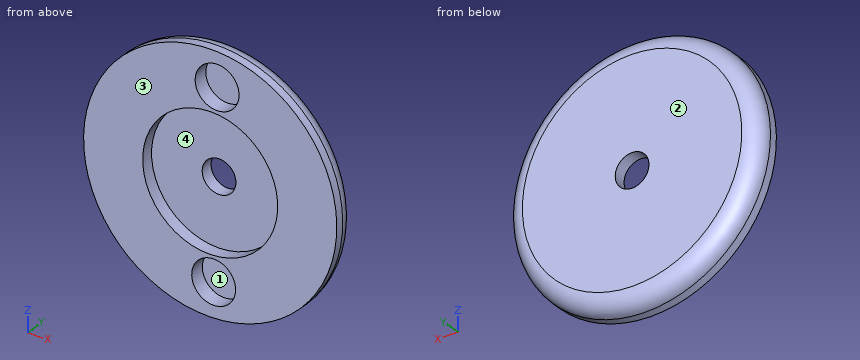
```python
from build123d import *

# Parameters (mm, degrees)
SKETCH2_W          = 15
SKETCH2_H          = 3
SKETCH3_R          = 8
CUT_EXTRUDE1_DEPTH = 1.5
CUT_EXTRUDE2_DEPTH = 1.5
SKETCH5_R          = 2.6
CUT_EXTRUDE3_DEPTH = 1.8
FILLET1_R          = 2


with BuildPart() as part:
    # Sketch2 → Revolve1 (revolve)
    with BuildSketch(Plane.XY, mode=Mode.PRIVATE) as revolve1_sk:
        with Locations((7.5, 1.5)):
            Rectangle(SKETCH2_W, SKETCH2_H)
    revolve(revolve1_sk.sketch.rotate(Axis((0, 0, 0), (0, 1, 0)), 90), axis=Axis((0, 0, 0), (0, 1, 0)))

    # Sketch3 → Cut-Extrude1 (cut)
    with BuildSketch(Plane.XZ):
        with Locations(Location((0, 0, 0), (0, 0, 270))):
            Circle(SKETCH3_R)
    extrude(amount=-CUT_EXTRUDE1_DEPTH, mode=Mode.SUBTRACT)

    # Sketch4 → Cut-Extrude2 (cut)
    with BuildSketch(Plane.XZ.offset(-1.5)):
        with BuildLine():
            ThreePointArc((0, -2), (2, 0), (0, 2))
            ThreePointArc((0, 2), (-2, 0), (0, -2))
        make_face()
    extrude(amount=-CUT_EXTRUDE2_DEPTH, mode=Mode.SUBTRACT)

    # Sketch5 → Cut-Extrude3 (cut)
    with BuildSketch(Plane.XZ):
        with Locations(Location((0.41, -10.964999997, 0), (0, 0, 270))):
            Circle(SKETCH5_R)
        with Locations(Location((0.82, 10.965000003, 0), (0, 0, 270))):
            Circle(SKETCH5_R)
    extrude(amount=-CUT_EXTRUDE3_DEPTH, mode=Mode.SUBTRACT)

    # Fillet1
    fillet1_edges = [part.edges().sort_by_distance(p)[0] for p in [
        (0, 3, 15),
    ]]
    fillet(fillet1_edges, radius=FILLET1_R)


solid = part.part
```
The listing builds one solid part. Answer for the finished solid, in the listing's coordinates (mm). Face numbers are marked on the shaded views. A direction names the side the tool comes from. Give positions to 0.01 mm unless a question says otherwise; leave off trailing zeros. Order: outer loops, then holes, each group sorted by start corner. A loop starts at its lowest first (then second) coordinate and runs counter-clockwise, first axis right, second up.
1) Find section C-C on y = 0.65. Write down the section's boundary in (x, z) (3 decimals), then the cut area to 3 significant figures.
Reported:
outline: circle Ø30 at (0, 0); hole circle Ø16 at (0, 0); hole circle Ø5.2 at (0.41, -10.965); hole circle Ø5.2 at (0.82, 10.965)
area: 463 mm2
2) Find section B-B on x = 0. Write down the section's boundary in (y, z).
Reported:
outline: (0, -15) - (1, -15) arc R2 ccw to (3, -13) - (3, -2) - (1.5, -2) - (1.5, -8) - (0, -8) - (0, -8.4) - (1.8, -8.4) - (1.8, -13.53) - (0, -13.53) - close; (0, 8) - (1.5, 8) - (1.5, 2) - (3, 2) - (3, 13) arc R2 ccw to (1, 15) - (0, 15) - (0, 13.43) - (1.8, 13.43) - (1.8, 8.5) - (0, 8.5) - close
3) Determine the mould class of the marked faces 3 and 4 for opening direction X: pulls with the +X half, pulls with the -X half, needs draft (parallel to the pull), parting line crosses it, or undercut.
Reported:
face 3: needs draft
face 4: undercut
4) Given P1, Ø4.5, axis at x = 0.82, z = 10.965, coming from the -Y side; P2, Ø5, axis at x = 0, z = 0, coming from the -Y side; P3, Ø1.5, axis at y = 2.5, z = 5.5, coming from the +X side, each flat-ended and moving along its own axis, determine where each tip first touches the part or whether it passes through.
Reported:
P1: stops at y = 1.8
P2: stops at y = 1.5
P3: stops at x = 13.9
5) Consider line 1 along X through (y, z) = (0.4, 0); line 2 along Y through (x, z) = (5.5, 4); line 3 along X through (y, z) = (1.1, 2.5). Determine where each line is inside the solid, lowest interval first.
Reported:
line 1: x = -15 to -8, 8 to 15
line 2: y = 1.5 to 3
line 3: x = -14.79 to -7.6, 7.6 to 14.79
6) For the marked faces 1 and 2, determine the directions among +Z, -Z, +X, -X, +Y, -Y from which every point of the face is accessible in a straight line to the end or side of a thin tool.
Reported:
face 1: -Y
face 2: +Z, -Z, +X, -X, +Y
7) Find section A-A on z = 0. Write down the section's boundary in (x, y), then the cut area to 3 significant figures.
Reported:
outline: (-15, 0) - (-8, 0) - (-8, 1.5) - (-2, 1.5) - (-2, 3) - (-13, 3) arc R2 ccw to (-15, 1) - close; (2, 1.5) - (8, 1.5) - (8, 0) - (15, 0) - (15, 1) arc R2 ccw to (13, 3) - (2, 3) - close
area: 58.3 mm2
